For this review, take the finished solid that the model builds, in its own axes (mm). Give positions to 0.01 mm unless a question says otherwise; leave off trailing zeros. Write each loop counter-clockwise with the first axis right and the second up, starting at its lowest first coordinate (ties: lowest second). Pieces come first, ordered by that corner, then holes. Notation, with made-up numbers: M 35.5,-7.5 L 47.5,-7.5 A21 ccw 47.5,9.5 Z; hole C -2,26.5 d7. An arc over 180 degrees is marked long. Use one line per item in the form item = value. Start each with the question number.
Q1. Mouldability with a two-part tool opening along X and no side actions: class faces 1 (the flat face through (-25, 0, 1)), 2 (the cylindrical face through (2.817, 21.768, 0.76)), 3 (the flat face through (0, 0, 0)) as released by +X, released by -X, zero draft, split by the parting line, or undercut.
Q2. Clearance check with flat-ended pins moving along their axes: pin 1 Ø0.9 at (x, y) = (-7.26, 22.5) entering from +Z; pin 2 Ø1.7 at (x, y) = (-12.38, 22.5) entering from -Z. State where each tip first meets the part, or that it passes through.
Q3. Consider section A-A on x = -9.82. Write out the cut boundary in (y, z), and give its area (3 significant figures).
Q4. For probe 1 along Y at (x, z) = (-9.82, 1.15); probe 2 along Y at (x, z) = (-14.5, 0.6), list the stretches that pass through material, from the lowest coordinate up. Write a range as [from, to].
Q5. Consider section D-D on x = -2. Write out the cut boundary in (y, z), and give its area (3 significant figures).
Q6. Consider section B-B on z = 0.4. Give the number of separate pieces and of enclosed holes in the cut face, and give its area (3 significant figures).
```python
from build123d import *

# Parameters (mm, degrees)
SKETCH1_W           = 50
SKETCH1_H           = 50
BOSS_EXTRUDE1_DEPTH = 1.5
SKETCH2_R           = 0.75
CUT_EXTRUDE1_DEPTH  = 2.5


with BuildPart() as part:
    # Sketch1 → Boss-Extrude1 (new body)
    with BuildSketch(Plane.XY):
        Rectangle(SKETCH1_W, SKETCH1_H)
    extrude(amount=BOSS_EXTRUDE1_DEPTH)

    # Sketch2 → Cut-Extrude1 (cut, through all)
    with BuildSketch(Plane.XY.offset(1.5)):
        with Locations((-17.5, -22.5)):
            Circle(SKETCH2_R)
        with Locations((-14.94, -22.5)):
            Circle(SKETCH2_R)
        with Locations((-12.38, -22.5)):
            Circle(SKETCH2_R)
        with Locations((-9.82, -22.5)):
            Circle(SKETCH2_R)
        with Locations((-7.26, -22.5)):
            Circle(SKETCH2_R)
        with Locations((-4.7, -22.5)):
            Circle(SKETCH2_R)
        with Locations((-2.14, -22.5)):
            Circle(SKETCH2_R)
        with Locations((0.42, -22.5)):
            Circle(SKETCH2_R)
        with Locations((2.98, -22.5)):
            Circle(SKETCH2_R)
        with Locations((5.54, -22.5)):
            Circle(SKETCH2_R)
        with Locations((8.1, -22.5)):
            Circle(SKETCH2_R)
        with Locations((10.66, -22.5)):
            Circle(SKETCH2_R)
        with Locations((13.22, -22.5)):
            Circle(SKETCH2_R)
        with Locations((15.78, -22.5)):
            Circle(SKETCH2_R)
        with Locations((18.34, -22.5)):
            Circle(SKETCH2_R)
        with Locations((18.34, 22.5)):
            Circle(SKETCH2_R)
        with Locations((15.78, 22.5)):
            Circle(SKETCH2_R)
        with Locations((13.22, 22.5)):
            Circle(SKETCH2_R)
        with Locations((10.66, 22.5)):
            Circle(SKETCH2_R)
        with Locations((8.1, 22.5)):
            Circle(SKETCH2_R)
        with Locations((5.54, 22.5)):
            Circle(SKETCH2_R)
        with Locations((2.98, 22.5)):
            Circle(SKETCH2_R)
        with Locations((0.42, 22.5)):
            Circle(SKETCH2_R)
        with Locations((-2.14, 22.5)):
            Circle(SKETCH2_R)
        with Locations((-4.7, 22.5)):
            Circle(SKETCH2_R)
        with Locations((-7.26, 22.5)):
            Circle(SKETCH2_R)
        with Locations((-9.82, 22.5)):
            Circle(SKETCH2_R)
        with Locations((-12.38, 22.5)):
            Circle(SKETCH2_R)
        with Locations((-14.94, 22.5)):
            Circle(SKETCH2_R)
        with Locations((-17.5, 22.5)):
            Circle(SKETCH2_R)
    extrude(amount=-CUT_EXTRUDE1_DEPTH, mode=Mode.SUBTRACT)


solid = part.part
```
Working result:
q1.face_1 = released by -X
q1.face_2 = undercut
q1.face_3 = zero draft
q2.pin_1 = through
q2.pin_2 = 0
q3.outline = M -25,0 L -23.25,0 L -23.25,1.5 L -25,1.5 Z; M -21.75,0 L 21.75,0 L 21.75,1.5 L -21.75,1.5 Z; M 23.25,0 L 25,0 L 25,1.5 L 23.25,1.5 Z
q3.area = 70.5 mm²
q4.probe_1 = [-25, -23.25], [-21.75, 21.75], [23.25, 25]
q4.probe_2 = [-25, -23.11], [-21.89, 21.89], [23.11, 25]
q5.outline = M -25,0 L -23.24,0 L -23.24,1.5 L -25,1.5 Z; M -21.76,0 L 21.76,0 L 21.76,1.5 L -21.76,1.5 Z; M 23.24,0 L 25,0 L 25,1.5 L 23.24,1.5 Z
q5.area = 70.6 mm²
q6.separate_pieces = 1
q6.enclosed_holes = 30
q6.area = 2,450 mm²
